Build history of the part. All positions in model axes, mm. A direction names the side the tool comes from. Coordinates: 2 decimals unless noted, no trailing zeros. Loops run counter-clockwise (first coordinate to the right, second up) from the corner with the lowest first, then second, coordinate; pieces in that order, holes last.
Item 1: Drill centre lines: line 1 along X through (y, z) = (-3, 12.5); line 2 along Y through (x, z) = (7.5, -17) (3 decimals); line 3 along X through (y, z) = (0.25, 9.5). Where is each one in solid material? Low to high.
Item 2: Cut at C-C (y = -1.25). List the corners of the cut face in (x, z).
Item 3: 3-axis set-ups, long thin cutter, end or side, ignore diameter. For faces 1 (the face through (51.302, -0.065, -0.395)), 2 (the face through (-40.142, 1.654, 0.625)): which of +Z, -Z, +X, -X, +Y, -Y reach the whole face in a straight line?
Item 4: Mould opens along X. For faces 3 (the face through (-16, -3.175, 29)), 4 (the face through (0.74, -0.07, 26.92)), 5 (the face through (52.701, 1.364, -0.423)) say: released by +X, released by -X, zero draft, split by the parting line, or undercut.
Item 5: Flat gauge pins, fed straight in: pin 1 (1.5 mm diameter, centred on y = -2, z = 13.5, fed in from -X); pin 2 (3 mm diameter, centred on x = -10, z = -20, fed in from -Y) (3 decimals); pin 3 (2 mm diameter, centred on y = 0.5, z = -1, fed in from +X); pin 4 (2.5 mm diameter, centred on x = 41.65, z = 0, fed in from +Y) (1 decimal). Where does each tip first touch, or does it go through?
from build123d import *

# Parameters (mm, degrees)
SKETCH2_W                                         = 109.22
SKETCH2_H                                         = 60.452
BOSS_EXTRUDE1_DEPTH                               = 3.175
FILLET3_R                                         = 6.35
SHELL1_T                                          = -2
CSK_FOR_4_FLAT_HEAD_MACHINE_SCREW_100_D           = 3.2639
CSK_FOR_4_FLAT_HEAD_MACHINE_SCREW_100_CSINK_D     = 5.715
CSK_FOR_4_FLAT_HEAD_MACHINE_SCREW_100_CSINK_ANGLE = 100


with BuildPart() as part:
    # Sketch2 → Boss-Extrude1 (new, symmetric)
    with BuildSketch(Plane(origin=(0, 0, 0), x_dir=(1, 0, 0), z_dir=(0, 1, 0))):
        Rectangle(SKETCH2_W, SKETCH2_H)
    extrude(amount=BOSS_EXTRUDE1_DEPTH, both=True)

    # Fillet3
    fillet3_edges = [part.edges().sort_by_distance(p)[0] for p in [
        (-54.61, 3.175, 0),
        (0, 3.175, -30.226),
        (54.61, 3.175, 0),
        (0, 3.175, 30.226),
    ]]
    fillet(fillet3_edges, radius=FILLET3_R - 0.0001)  # a hair under: the kernel refuses the full size

    # Shell1
    shell1_openings = [part.faces().sort_by_distance(p)[0] for p in [
        (0, -3.175, 0),
    ]]
    offset(amount=SHELL1_T, openings=shell1_openings)

    # CSK for #4 Flat Head Machine Screw (100)1 (through all)
    with Locations(Plane(origin=(0, 3.175, 0), x_dir=(1, 0, 0), z_dir=(0, 1, 0))):
        with Locations((41.65, 0)):
            csk_for_4_flat_head_machine_screw_100 = CounterSinkHole(CSK_FOR_4_FLAT_HEAD_MACHINE_SCREW_100_D / 2, CSK_FOR_4_FLAT_HEAD_MACHINE_SCREW_100_CSINK_D / 2, counter_sink_angle=CSK_FOR_4_FLAT_HEAD_MACHINE_SCREW_100_CSINK_ANGLE)

    # Mirror1: CSK for #4 Flat Head Machine Screw (100)1 across plane
    add(csk_for_4_flat_head_machine_screw_100.mirror(Plane(origin=(0, 0, 0), x_dir=(0, 0, 1), z_dir=(1, 0, 0))), mode=Mode.SUBTRACT)


solid = part.part
Filled sheet:
1. line 1: x = -54.61 to -52.61, 52.61 to 54.61
1. line 2: y = 1.175 to 3.175
1. line 3: x = -53.61 to -50.94, 50.94 to 53.61
2. outline: (-54.31, -29.93) - (54.31, -29.93) - (54.31, 29.93) - (-54.31, 29.93) - close; hole (-52.16, -27.78) - (52.16, -27.78) - (52.16, 27.78) - (-52.16, 27.78) - close
3. face 1: -Y
3. face 2: +Y, -Y
4. face 3: zero draft
4. face 4: undercut
4. face 5: released by +X
5. pin 1: stops at x = -54.6
5. pin 2: stops at y = 1.175
5. pin 3: stops at x = 54.02
5. pin 4: passes through
